Design review of the part shown in the three views and the two pictorial views. Dimensions are in mm from the part's minimum x, y and z. A direction names the side the tool comes from. Give positions to 0.01 mm unless a question says otherwise; leave off trailing zeros. Loops run counter-clockwise (first coordinate to the right, second up) from the corner with the lowest first, then second, coordinate; pieces in that order, holes last.
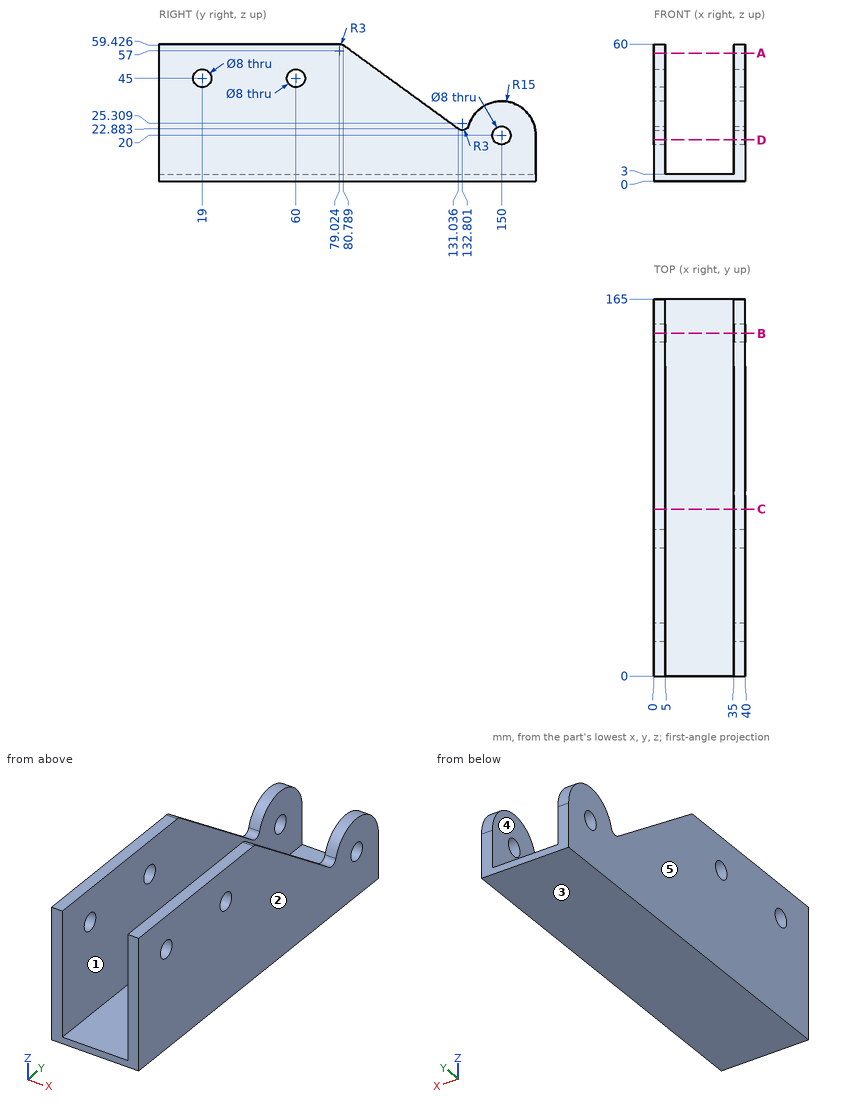
Q1. Mouldability with a two-part tool opening along X and no side actions: class the marked faces 3, 4 and 5 as +X half, -X half, draft (parallel to the pull), parting line (faces both ways), or undercut.
Answers:
face 3: draft
face 4: undercut
face 5: -X half
Q2. Machinability: for the marked faces 1 and 2, which of the approach directions +Z, -Z, +X, -X, +Y, -Y give a long, thin tool a straight path to every point of the face, cutting with its end or side? Answer none if there is none.
Answers:
face 1: +Z, +Y, -Y
face 2: +Z, -Z, +X, +Y, -Y
Q3. Consider section D-D on z = 18. Give the boundary of the cut face in (x, y) (1 decimal).
Answers:
outline: (0, 0) - (5, 0) - (5, 146.5) - (0, 146.5) - close; (0, 153.5) - (5, 153.5) - (5, 165) - (0, 165) - close; (35, 0) - (40, 0) - (40, 146.5) - (35, 146.5) - close; (35, 153.5) - (40, 153.5) - (40, 165) - (35, 165) - close
Q4. For pin 1 Ø6.5 at (y, z) = (19, 45) entering from +X; pin 2 Ø5 at (x, y) = (24.5, 26) entering from +Z, all flat-tipped, find the tip position at first contact; note any pin that passes through.
Answers:
pin 1: passes through
pin 2: stops at z = 3
Q5. Consider section A-A on z = 56. Give the boundary of the cut face in (x, y).
Answers:
outline: (0, 0) - (5, 0) - (5, 85.5) - (0, 85.5) - close; (35, 0) - (40, 0) - (40, 85.5) - (35, 85.5) - close
Q6. For probe 1 along X at (y, z) = (147.5, 9.5); probe 2 along Y at (x, z) = (38, 45) (1 decimal); probe 3 along Z at (x, y) = (2, 150), list the stretches that pass through material, from the lowest coordinate up.
Answers:
probe 1: x = 0 to 5, 35 to 40
probe 2: y = 0 to 15, 23 to 56, 64 to 100.6
probe 3: z = 0 to 16, 24 to 35
Q7. Consider section B-B on y = 150. Give the boundary of the cut face in (x, z), plus the area to 3 significant figures.
Answers:
outline: (0, 0) - (40, 0) - (40, 16) - (35, 16) - (35, 3) - (5, 3) - (5, 16) - (0, 16) - close; (0, 24) - (5, 24) - (5, 35) - (0, 35) - close; (35, 24) - (40, 24) - (40, 35) - (35, 35) - close
area: 360 mm2
Q8. Consider section C-C on y = 73. Give the boundary of the cut face in (x, z).
Answers:
outline: (0, 0) - (40, 0) - (40, 60) - (35, 60) - (35, 3) - (5, 3) - (5, 60) - (0, 60) - close
